from build123d import *

# Parameters (mm, degrees)
SKETCH1_W           = 38.1
SKETCH1_H           = 88.9
BOSS_EXTRUDE1_DEPTH = 1143
SKETCH2_R           = 22.225
CUT_EXTRUDE4_DEPTH  = 918.6545
SKETCH3_R           = 4.7625
CUT_EXTRUDE5_DEPTH  = 1145.498323502
FILLET1_R           = 3.175


with BuildPart() as part:
    # Sketch1 → Boss-Extrude1 (new body)
    with BuildSketch(Plane(origin=(0, 0, 0), x_dir=(1, 0, 0), z_dir=(0, 1, 0))):
        Rectangle(SKETCH1_W, SKETCH1_H)
    extrude(amount=BOSS_EXTRUDE1_DEPTH)

    # Sketch2 → Cut-Extrude4 (cut)
    with BuildSketch(Plane(origin=(19.05, 0, 0), x_dir=(0, 0, -1), z_dir=(1, 0, 0))):
        with Locations((12.7, 458.7875)):
            Circle(SKETCH2_R)
        with Locations((12.7, 939.8)):
            Circle(SKETCH2_R)
    extrude(amount=-CUT_EXTRUDE4_DEPTH, mode=Mode.SUBTRACT)

    # Sketch3 → Cut-Extrude5 (cut, through all)
    with BuildSketch(Plane(origin=(19.05, 0, 0), x_dir=(0, 0, -1), z_dir=(1, 0, 0))):
        with Locations((-33.3375, 112.7125)):
            Circle(SKETCH3_R)
        with Locations((-33.3375, 608.0125)):
            Circle(SKETCH3_R)
        with Locations((-33.3375, 1103.3125)):
            Circle(SKETCH3_R)
    extrude(amount=-CUT_EXTRUDE5_DEPTH, mode=Mode.SUBTRACT)

    # Fillet1
    fillet1_edges = [part.edges().sort_by_distance(p)[0] for p in [
        (19.05, 571.5, 44.45),
        (-19.05, 571.5, 44.45),
        (-19.05, 571.5, -44.45),
        (19.05, 571.5, -44.45),
    ]]
    fillet(fillet1_edges, radius=FILLET1_R)


solid = part.part
Geometry check sheet. Reference: the model listing, model coordinates, mm. Round coordinates to 2 decimals unless told otherwise and drop trailing zeros. Loops run counter-clockwise (first coordinate to the right, second up) from the corner with the lowest first, then second, coordinate; pieces in that order, holes last. Notation, with made-up numbers: (40.5, 86.25) - (44.5, 86.25) arc R21 ccw to (44.5, 90.25) - close; hole circle Ø11 at (30.25, 53.25). An arc over 180 degrees is marked (long way). One line per question, with ' | ' between items. Start each with the question number.
1. Cross-section at B-B on y = 939.8. Record the cut outline in (x, z) (3 decimals).
2. Draft check along Y on faces 1 (the face through (0, 563, 44.45)), 2 (the face through (0.27, 437.09, -7.88)), 3 (the face through (0, 0, -1)), 4 (the face through (0.267, 961.836, -9.807)). Enter one of: released by +Y, released by -Y, zero draft, split by the parting line, or undercut.
3. Scan lines: line 1 (Y direction, x = 1.5, z = -12.7) (1 decimal); line 2 (Y direction, x = -12, z = -21); line 3 (Y direction, x = 14, z = 35). Record each from-to range of solid material in increasing order. Write a range as [from, to].
4. Depth check by flat-ended pin: pin 1 (5.5 mm diameter, centred on y = 112.71, z = 33.34, fed in from -X). Enter the tip coordinate at first touch or a pass-through.
5. Cross-section at A-A on z = -12.7. State how many separate pieces and enclosed holes the cut face has, then the cut area to 3 significant figures.
Taken from the geometry:
1) outline: (-19.05, -41.275) arc R3.175 ccw to (-15.875, -44.45) - (15.875, -44.45) arc R3.175 ccw to (19.05, -41.275) - (19.05, -34.925) - (-19.05, -34.925) - close; (-19.05, 9.525) - (19.05, 9.525) - (19.05, 41.275) arc R3.175 ccw to (15.875, 44.45) - (-15.875, 44.45) arc R3.175 ccw to (-19.05, 41.275) - close
2) face 1: zero draft | face 2: undercut | face 3: released by -Y | face 4: undercut
3) line 1: [0, 436.6], [481, 917.6], [962, 1143] | line 2: [0, 438.17], [479.4, 919.18], [960.42, 1143] | line 3: [0, 108.25], [117.18, 603.55], [612.48, 1098.85], [1107.78, 1143]
4) pin 1: through
5) separate pieces: 3 | enclosed holes: 0 | area: 40,200 mm²
